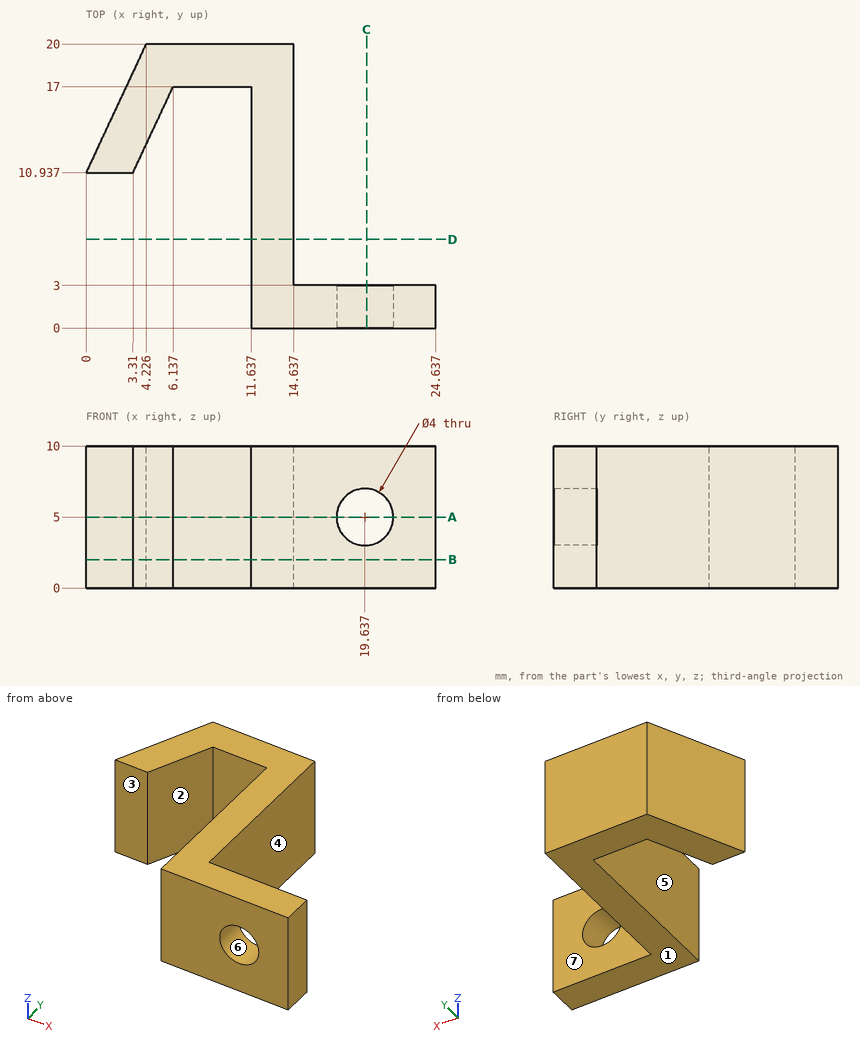
Part print with two shaded views. Sizes in mm from the minimum x, y, z corner. A direction names the side the tool comes from. Coordinates: 2 decimals unless noted, no trailing zeros. Write each loop counter-clockwise with the first axis right and the second up, starting at its lowest first coordinate (ties: lowest second). Pieces come first, ordered by that corner, then holes. Notation, with made-up numbers: (-17, 49.25) - (38, 49.25) arc R20 cw to (38, 81.25) - close; hole circle Ø6 at (-22, -20.5). An arc over 180 degrees is marked (long way). One line per item, written item: value. Start each with the question number.
1. Slice it at D-D (y = 6.25). Write the cut outline in (x, z).
2. Mould opens along X. For the marked faces 4, 5, 6 and 7 say: released by +X, released by -X, zero draft, split by the parting line, or undercut.
3. Slice it at A-A (z = 5). Write the cut outline in (x, y).
4. Probe line 1 (X direction, y = 9.25, z = 6.25); line 2 (Y direction, x = 11.5, z = 9); line 3 (X direction, y = 2.5, z = 2.75). List the from-to ranges inside material, lowest first. Write a range as from..to.
5. Slice it at B-B (z = 2). Write the cut outline in (x, y), plus the area to 3 significant figures.
6. Slice it at C-C (x = 19.75). Write the cut outline in (y, z), plus the area to 3 significant figures.
7. Tool access for the marked faces 1, 2 and 3: list every direction of +Z, -Z, +X, -X, +Y, -Y with a clear straight run to the whole face (end or side of a thin tool).
8. Flat gauge pins, fed straight in: pin 1 (3 mm diameter, centred on y = 12.5, z = 5.5, fed in from -X); pin 2 (3 mm diameter, centred on x = 9.5, z = 7.5, fed in from -Y); pin 3 (3 mm diameter, centred on y = 5.5, z = 5.5, fed in from -X). Where does each tip first touch, or does it go through?
Answers below:
1. outline: (11.64, 0) - (14.64, 0) - (14.64, 10) - (11.64, 10) - close
2. face 4: released by +X
2. face 5: undercut
2. face 6: undercut
2. face 7: zero draft
3. outline: (0, 10.94) - (3.31, 10.94) - (6.14, 17) - (11.64, 17) - (11.64, 0) - (17.64, 0) - (17.64, 3) - (14.64, 3) - (14.64, 20) - (4.23, 20) - close; (21.64, 0) - (24.64, 0) - (24.64, 3) - (21.64, 3) - close
4. line 1: x = 11.64..14.64
4. line 2: y = 17..20
4. line 3: x = 11.64..24.64
5. outline: (0, 10.94) - (3.31, 10.94) - (6.14, 17) - (11.64, 17) - (11.64, 0) - (24.64, 0) - (24.64, 3) - (14.64, 3) - (14.64, 20) - (4.23, 20) - close
5. area: 134 mm^2
6. outline: (0, 0) - (3, 0) - (3, 3) - (0, 3) - close; (0, 7) - (3, 7) - (3, 10) - (0, 10) - close
6. area: 18.0 mm^2
7. face 1: -Z, +X, -X, +Y, -Y
7. face 2: +Z, -Z, -Y
7. face 3: +Z, -Z, -X, -Y
8. pin 1: stops at x = 0.03
8. pin 2: stops at y = 17
8. pin 3: stops at x = 11.64
